Source: CAD feature listing. Evaluate the final solid. Frame: model axes, mm. A direction names the side the tool comes from. Coordinates: 2 decimals unless noted, no trailing zeros. Order: outer loops, then holes, each group sorted by start corner. A loop starts at its lowest first (then second) coordinate and runs counter-clockwise, first axis right, second up. Notation, with made-up numbers: (8, 63.5) -> (46, 63.5) arc R27 ccw to (46, 82.5) -> close; hole circle Ø1 at (-29.75, -12.5). An arc over 180 degrees is marked (long way). Write item = value, one per line. Start each with the question number.
Item 1: Set-up query: faces 1 (the flat face through (0, 2.5, 0)), 2 (the cylindrical face through (-2, -21, 0)). Return all of +Z, -Z, +X, -X, +Y, -Y with unobstructed straight access to the full face (end or side cutting, diameter ignored); none if empty.
Item 2: Contact query for flat-ended pins moving along their axis: pin 1 (3 mm diameter, centred on y = -33.5, z = 5, fed in from +X); pin 2 (8 mm diameter, centred on x = -2, y = -17, fed in from +Z); pin 3 (7 mm diameter, centred on x = -2.5, z = 1, fed in from -Y); pin 4 (6 mm diameter, centred on x = 4.5, y = -34.5, fed in from +Z). Output: stop coordinate, or through.
Item 3: Ray query, line 1 along Z through (x, y) = (-2, 1); line 2 along Y through (x, z) = (2.5, -2); line 3 along Y through (x, z) = (1.25, 3.25). Return the intervals inside material, ascending. Write a range as [from, to].
Item 4: Section query A-A (y = -17). Output: boundary loops of the cut face in (x, z).
```python
from build123d import *

# Parameters (mm, degrees)
SKETCH_19_R     = 2
EXTRUDE_1_DEPTH = 42
CHAMFER_1_SIZE  = 1


with BuildPart() as part:
    # 草图16 → 旋转1 (revolve)
    with BuildSketch(Plane.XY):
        with BuildLine():
            Line((0, 0), (-7, 0))
            add(Edge.make_bspline(
                [(-2, 2.5), (-4.820865147, 1.972200791), (-7, 0)],
                knots=[0, 0, 0, 1, 1, 1], degree=2))
            Line((-2, 2.5), (0, 2.5))
            Line((0, 2.5), (0, 0))
        make_face()
    revolve(axis=Axis((0, 0, 0), (0, 1, 0)))

    # 草图19 → 凸台-拉伸1 (add)
    with BuildSketch(Plane(origin=(0, 0, 0), x_dir=(1, 0, 0), z_dir=(0, 1, 0))):
        with Locations(Location((0, 0, 0), (0, 0, 270))):
            Circle(SKETCH_19_R)
    extrude(amount=-EXTRUDE_1_DEPTH)

    # 倒角1
    chamfer_1_edges = [part.edges().sort_by_distance(p)[0] for p in [
        (0, -42, -2),
        (0, 0, -2),
    ]]
    chamfer(chamfer_1_edges, length=CHAMFER_1_SIZE)


solid = part.part
```
Computed:
q1.face_1 = +Z, -Z, +X, -X, +Y
q1.face_2 = -Y
q2.pin_1 = through
q2.pin_2 = 2
q2.pin_3 = -42
q2.pin_4 = 1.32
q3.line_1 = [-5.35, 5.35]
q3.line_2 = [0, 2.2]
q3.line_3 = [0, 2.11]
q4.outline = circle Ø4 at (0, 0)
